Autodesk Inventor part; units mm, degrees
ref_plane "YZ Plane" through (0, 0, 0) normal (1, 0, 0) x (0, 1, 0)
ref_plane "XZ Plane" through (0, 0, 0) normal (0, 1, 0) x (-1, 0, 0)
ref_plane "XY Plane" through (0, 0, 0) normal (0, 0, 1) x (1, 0, 0)
sketch "Sketch1" plane through (0, 0, 0) normal (0, 0, 1) x (1, 0, 0)
  line L0 (4.9734, -6.5186) -> (-5.17, -6.5186) construction
  line L1 (-5.1132, 9.4814) -> (-5.1132, 4.4814)
  line L2 (-5.1132, -2.5186) -> (4.8868, -2.5186)
  line L3 (4.8868, 9.4814) -> (2.8868, 9.4814)
  line L4 (2.8868, 9.4814) -> (1.5056, 7.4814)
  arc A0 (-1.9585, 7.4814) -> (1.5056, 7.4814) centre (-0.2265, 8.4814) ccw
  line L5 (-1.9585, 7.4814) -> (-3.1132, 9.4814)
  line L6 (-3.1132, 9.4814) -> (-5.1132, 9.4814)
  line L7 (4.8868, 9.4814) -> (4.8868, -2.5186)
  line L8 (-5.1132, 4.4814) -> (-17.1132, 4.4814)
  line L9 (-17.1132, 4.4814) -> (-17.1132, -2.5186)
  line L10 (-17.1132, -2.5186) -> (-5.1132, -2.5186)
  dimension "d28" = 2
  dimension "d29" = 120
  dimension "d30" = 12
  dimension "d31" = 10
  dimension "d32" = 4
  dimension "d33" = 2
  dimension "d34" = 2
  dimension "d35" = 2
  dimension "d36" = 2
  dimension "d45" = 12
  dimension "d48" = 11
revolve "Revolution1" add sketch "Sketch1" angle 360 about axis through (4.9734, -6.5186, 0) along (-1, 0, 0)
sketch "Sketch3" plane through (4.8868, -6.5186, 0) normal (1, 0, 0) x (0, 0, -1)
  circle A0 centre (0, 0) radius 4
  line L0 (0, 0) -> (-8, 0) construction
  point P0 (0, 6.5186)
  point P1 (0, -8)
  point P2 (8, 0)
  point P3 (0, 8)
  dimension "d49" = 8
  dimension "d52" = 360
hole "Hole2" at (4.8868, -6.5186, 0) at (4.8868, -6.5186, 8) at (4.8868, -14.5186, 0) at (4.8868, -6.5186, -8) at (4.8868, 1.4814, 0) direction (-1, 0, 0) diameter 2.4 end through all counterbore diameter 4 counterbore depth 18
properties part number "motor_trinse"
Build history of the part. All positions in model axes, mm. A direction names the side the tool comes from. Round coordinates to 2 decimals unless told otherwise and drop trailing zeros. Loops run counter-clockwise (first coordinate to the right, second up) from the corner with the lowest first, then second, coordinate; pieces in that order, holes last.
Item 1: Saw through at B-B (z = 0). State how many separate pieces and enclosed holes the cut face has, then the cut area to 3 significant figures.
Item 2: Saw through at A-A (x = -11). List the corners of the cut face in (y, z).
Item 3: Saw through at C-C (x = -1.5). List the corners of the cut face in (y, z).
Item 4: Two-plate mould, pull along Z, no slides. Class faces 1 (the face through (-4.239, 3.434, 0.434)), 2 (the face through (-4.239, -12.566, 0.434)), 3 (the face through (-17.113, -7, 5)), 4 (the face through (-4.127, 0.864, 14.195)): released by +Z, released by -Z, zero draft, split by the parting line, or undercut.
Item 5: Pin check, flat tips, straight feed: P1, Ø1.5, axis at y = -1, z = 12, coming from the -X side; P2, Ø3, axis at y = 1.48, z = 0, coming from the +X side; P3, Ø4, axis at x = -14, y = -17.5, coming from the -Z side. Stop position of each tip, or through.
Item 6: Drill centre lines: line 1 along Y through (x, z) = (0, 0); line 2 along Z through (x, y) = (-6, -5); line 3 along Z through (x, y) = (-2.25, -10). Where is each one in solid material? Low to high.
Item 7: Which spindle directions (+Z, -Z, +X, -X, +Y, -Y) get a long thin tool onto all of the face, cutting with end or side? Do faces 5 (the face through (-13.113, -13, 0)), 6 (the face through (-5.113, 4, -4)), 7 (the face through (-15.14, -6.57, -6.8)), 8 (the face through (1.59, 0, -12.53)). Say none if no direction does.
Worked answers:
1. separate pieces: 4
1. enclosed holes: 0
1. area: 221 mm2
2. outline: circle Ø22 at (-6.52, 0); hole circle Ø4 at (-14.52, 0); hole circle Ø8 at (-6.52, 0); hole circle Ø4 at (-6.52, -8); hole circle Ø4 at (-6.52, 8); hole circle Ø4 at (1.48, 0)
3. outline: circle Ø26.92 at (-6.52, 0); hole circle Ø4 at (-14.52, 0); hole circle Ø8 at (-6.52, 0); hole circle Ø4 at (-6.52, -8); hole circle Ø4 at (-6.52, 8); hole circle Ø4 at (1.48, 0)
4. face 1: undercut
4. face 2: undercut
4. face 3: zero draft
4. face 4: split by the parting line
5. P1: stops at x = -5.11
5. P2: stops at x = -13.11
5. P3: stops at z = -6.35
6. line 1: y = -19.53 to -16.52, -12.52 to -10.52, -2.52 to -0.52, 3.48 to 6.49
6. line 2: z = -10.89 to -9.3, -6.7 to -3.7, 3.7 to 6.7, 9.3 to 10.89
6. line 3: z = -14.08 to -1.97, 1.97 to 14.08
7. face 5: +X
7. face 6: -X
7. face 7: +X, -X
7. face 8: none
